Autodesk Inventor part; units mm, degrees
ref_plane "YZ Plane" through (0, 0, 0) normal (1, 0, 0) x (0, 1, 0)
ref_plane "XZ Plane" through (0, 0, 0) normal (0, 1, 0) x (-1, 0, 0)
ref_plane "XY Plane" through (0, 0, 0) normal (0, 0, 1) x (1, 0, 0)
sketch "Sketch1" plane through (0, 0, 0) normal (0, 0, 1) x (1, 0, 0)
  line L0 (3, 125) -> (32, 125)
  line L1 (32, 125) -> (32, 70)
  line L2 (3, 82) -> (3, 125)
  line L3 (-16, 0) -> (96, 0)
  line L4 (32, 70) -> (69.5, 55)
  line L5 (69.5, 55) -> (75.9585, 55)
  line L6 (80, 48) -> (80, 47)
  line L7 (80, 47) -> (5.6083, 47)
  line L8 (3, 82) -> (0, 79)
  line L9 (0, 79) -> (0, 62)
  line L10 (80, 48) -> (75.9585, 55)
  line L11 (5.6083, 47) -> (0, 62)
  point P0 (0, 0)
  point P1 (80, 55)
  dimension "d0" = 29
  dimension "d1" = 250
  dimension "d7" = 94
  dimension "d8" = 158
  dimension "d9" = 140
  dimension "d10" = 135
  dimension "d11" = 3
  dimension "d19" = 15
  dimension "d12" = 37.5
  dimension "d13" = 110
  dimension "d14" = 77
  dimension "d15" = 30
  dimension "d16" = 1
  dimension "d17" = 20.5
  dimension "d18" = 124
revolve "Revolution1" add sketch "Sketch1" angle 360 about axis through (-10, 0, 0) along (1, 0, 0)
sketch "Sketch2" plane through (0, 0, 0) normal (1, 0, 0) x (0, 1, 0)
  circle A0 centre (0, 100) radius 13
  line L0 (0, 44.8) -> (0, 25.2) construction
  line L1 (-9.8, 0) -> (9.8, 0) construction
  dimension "d2" = 26
  dimension "d3" = 200
extrude "Extrusion1" cut sketch "Sketch2" along normal through all both and the other way through all
pattern_circular "Circular Pattern1" count 8 over 360 about axis through (-10, 0, 0) along (1, 0, 0) of "Extrusion1"
equation "\"d2\" = d"
equation "\"d3\" = D1_"
equation "\"d0\" = b"
equation "\"d1\" = D_"
equation "\"d7\" = d1__"
equation "\"d8\" = D2_"
equation "\"d9\" = Dm"
equation "\"d11\" = h_"
equation "\"d12\" = 2.5 * d19"
equation "\"d13\" = Dn"
equation "\"d14\" = h4_"
equation "\"d18\" = D7_"
equation "\"b\" = 29"
equation "\"Dm\" = 140"
equation "\"D_\" = 250"
equation "\"D1_\" = 200"
equation "\"D2_\" = 158"
equation "\"d\" = 26"
equation "\"h_\" = 3"
equation "\"d1__\" = 94"
equation "\"h4_\" = 77"
equation "\"Dn\" = 110"
equation "\"D7_\" = 124"
properties part number "Flange 6-100-63 GOST 12821-80" material "Steel, Mild"
For this review, take the finished solid that the model builds, in its own axes (mm). A direction names the side the tool comes from. Round coordinates to 2 decimals unless told otherwise and drop trailing zeros. Order: outer loops, then holes, each group sorted by start corner. A loop starts at its lowest first (then second) coordinate and runs counter-clockwise, first axis right, second up. Notation, with made-up numbers: (62, 41.25) -> (75, 41.25) arc R9 ccw to (75, 55.25) -> close; hole circle Ø8 at (-30.5, -35). An arc over 180 degrees is marked (long way). Write item = value, one per line. Start each with the question number.
1) Insertion check: pin 1 (15.5 mm diameter, centred on y = 70.71, z = -70.71, fed in from +X); pin 2 (8 mm diameter, centred on y = -57, z = 56, fed in from +X); pin 3 (3 mm diameter, centred on x = 36, z = -59.5, fed in from +Y); pin 4 (3 mm diameter, centred on y = 87, z = -73, fed in from -X). Each pin has a flat end and moves straight along its axis. Give the tip position at first contact, or say it passes through.
2) Take a section at A-A on z = 0. Count the separate pieces of the cut face and the enclosed holes in it, plus the area to 3 significant figures.
3) The part is to be moulded in two halves that separate along Z. For faces 1 (the face through (17.3, -2.82, 112.69)), 2 (the face through (17.7, -124.88, 5.5)), 3 (the face through (3, 82, -26)), say which applies: +Z half, -Z half, draft (parallel to the pull), parting line (faces both ways), or undercut.
4) Take a section at C-C on z = 100. State the section outline as (x, y) points.
5) Tool access review of faces 4 (the face through (5.26, 45.72, -14.4)), 5 (the face through (32, 54, -54)): name each direction out of +Z, -Z, +X, -X, +Y, -Y from which nothing blocks a thin tool from reaching the whole face with its end or side.
6) To check wall thickness, follow line 1 (Z direction, x = 10, y = 0); line 2 (Y direction, x = 7, z = 5); line 3 (Z direction, x = 7, y = -73.5). State the ranges of each line that lie inside material, in increasing order. Write a range as from..to.
Verdict:
q1.pin_1 = through
q1.pin_2 = 32
q1.pin_3 = 36.51
q1.pin_4 = 3
q2.separate_pieces = 4
q2.enclosed_holes = 0
q2.area = 4,440 mm2
q3.face_1 = undercut
q3.face_2 = parting line
q3.face_3 = draft
q4.outline = (3, -75) -> (32, -75) -> (32, -13) -> (3, -13) -> close; (3, 13) -> (32, 13) -> (32, 75) -> (3, 75) -> close
q5.face_4 = -X
q5.face_5 = +X
q6.line_1 = -125..-113, -87..-47, 47..87, 113..125
q6.line_2 = -124.9..-112, -88..-46.73, 46.73..88, 112..124.9
q6.line_3 = -101.11..-83.41, -58.01..58.01, 83.41..101.11
